```python
from build123d import *

# Parameters (mm, degrees)
SKETCH1_W            = 130
SKETCH1_H            = 156
SKETCH1_R            = 3
BOSS_EXTRUDE1_DEPTH  = 10
SKETCH2_R            = 2.5
CUT_EXTRUDE1_DEPTH   = 10
SKETCH3_W            = 130
SKETCH3_H            = 10
BOSS_EXTRUDE2_DEPTH  = 10
SKETCH4_W            = 130
SKETCH4_H            = 10
BOSS_EXTRUDE3_DEPTH  = 10
SKETCH5_W            = 130
SKETCH5_H            = 10
CUT_EXTRUDE2_DEPTH   = 12.25
SKETCH6_W            = 130
SKETCH6_H            = 12.25
CUT_EXTRUDE3_DEPTH   = 20
SKETCH7_W            = 130
SKETCH7_H            = 10
BOSS_EXTRUDE5_DEPTH  = 2.25
SKETCH8_W            = 130
SKETCH8_H            = 10
BOSS_EXTRUDE6_DEPTH  = 2.25
SKETCH10_W           = 130
SKETCH10_H           = 10
BOSS_EXTRUDE8_DEPTH  = 10
SKETCH11_W           = 130
SKETCH11_H           = 10
BOSS_EXTRUDE10_DEPTH = 7
SKETCH12_W           = 130
SKETCH12_H           = 10
CUT_EXTRUDE4_DEPTH   = 7
SKETCH14_W           = 130
SKETCH14_H           = 10
CUT_EXTRUDE5_DEPTH   = 10


with BuildPart() as part:
    # Sketch1 → Boss-Extrude1 (new body)
    with BuildSketch(Plane(origin=(0, 0, 0), x_dir=(1, 0, 0), z_dir=(0, 1, 0))):
        with Locations((65, -43.506875339)):
            Rectangle(SKETCH1_W, SKETCH1_H)
        with Locations(Location((5, 27.493124661, 0), (0, 0, 270))):
            Circle(SKETCH1_R, mode=Mode.SUBTRACT)
        with Locations(Location((45, 27.493124661, 0), (0, 0, 270))):
            Circle(SKETCH1_R, mode=Mode.SUBTRACT)
        with Locations(Location((45, -12.506875339, 0), (0, 0, 270))):
            Circle(SKETCH1_R, mode=Mode.SUBTRACT)
        with Locations(Location((5, -12.506875339, 0), (0, 0, 270))):
            Circle(SKETCH1_R, mode=Mode.SUBTRACT)
        with Locations(Location((85, 27.493124661, 0), (0, 0, 270))):
            Circle(SKETCH1_R, mode=Mode.SUBTRACT)
        with Locations(Location((125, 27.493124661, 0), (0, 0, 270))):
            Circle(SKETCH1_R, mode=Mode.SUBTRACT)
        with Locations(Location((85, -12.506875339, 0), (0, 0, 270))):
            Circle(SKETCH1_R, mode=Mode.SUBTRACT)
        with Locations(Location((125, -12.506875339, 0), (0, 0, 270))):
            Circle(SKETCH1_R, mode=Mode.SUBTRACT)
        with Locations(Location((85, -74.506875339, 0), (0, 0, 270))):
            Circle(SKETCH1_R, mode=Mode.SUBTRACT)
        with Locations(Location((125, -74.506875339, 0), (0, 0, 270))):
            Circle(SKETCH1_R, mode=Mode.SUBTRACT)
        with Locations(Location((125, -114.506875339, 0), (0, 0, 270))):
            Circle(SKETCH1_R, mode=Mode.SUBTRACT)
        with Locations(Location((85, -114.506875339, 0), (0, 0, 270))):
            Circle(SKETCH1_R, mode=Mode.SUBTRACT)
        with Locations(Location((5, -74.506875339, 0), (0, 0, 270))):
            Circle(SKETCH1_R, mode=Mode.SUBTRACT)
        with Locations(Location((45, -74.506875339, 0), (0, 0, 270))):
            Circle(SKETCH1_R, mode=Mode.SUBTRACT)
        with Locations(Location((5, -114.506875339, 0), (0, 0, 270))):
            Circle(SKETCH1_R, mode=Mode.SUBTRACT)
        with Locations(Location((45, -114.506875339, 0), (0, 0, 270))):
            Circle(SKETCH1_R, mode=Mode.SUBTRACT)
    extrude(amount=BOSS_EXTRUDE1_DEPTH)

    # Sketch2 → Cut-Extrude1 (cut)
    with BuildSketch(Plane(origin=(0, 10, 0), x_dir=(1, 0, 0), z_dir=(0, 1, 0))):
        with Locations(Location((98, -31.506875339, 0), (0, 0, 270))):
            Circle(SKETCH2_R)
        with Locations(Location((98, -55.506875339, 0), (0, 0, 270))):
            Circle(SKETCH2_R)
        with Locations(Location((122, -55.506875339, 0), (0, 0, 270))):
            Circle(SKETCH2_R)
        with Locations(Location((122, -31.506875339, 0), (0, 0, 270))):
            Circle(SKETCH2_R)
    extrude(amount=-CUT_EXTRUDE1_DEPTH, mode=Mode.SUBTRACT)

    # Sketch3 → Boss-Extrude2 (add)
    with BuildSketch(Plane(origin=(0, 0, -34.493124661), x_dir=(-1, 0, 0), z_dir=(0, 0, -1))):
        with Locations((-65, 5)):
            Rectangle(SKETCH3_W, SKETCH3_H)
    extrude(amount=BOSS_EXTRUDE2_DEPTH)

    # Sketch4 → Boss-Extrude3 (add)
    with BuildSketch(Plane.XY.offset(121.506875339)):
        with Locations((65, 5)):
            Rectangle(SKETCH4_W, SKETCH4_H)
    extrude(amount=BOSS_EXTRUDE3_DEPTH)

    # Sketch5 → Cut-Extrude2 (cut)
    with BuildSketch(Plane.XY.offset(131.506875339)):
        with Locations((65, 5)):
            Rectangle(SKETCH5_W, SKETCH5_H)
    extrude(amount=-CUT_EXTRUDE2_DEPTH, mode=Mode.SUBTRACT)

    # Sketch6 → Cut-Extrude3 (cut)
    with BuildSketch(Plane(origin=(0, 10, 0), x_dir=(1, 0, 0), z_dir=(0, 1, 0))):
        with Locations((65, 38.368124661)):
            Rectangle(SKETCH6_W, SKETCH6_H)
    extrude(amount=-CUT_EXTRUDE3_DEPTH, mode=Mode.SUBTRACT)

    # Sketch7 → Boss-Extrude5 (add)
    with BuildSketch(Plane(origin=(0, 0, -32.243124661), x_dir=(-1, 0, 0), z_dir=(0, 0, -1))):
        with Locations((-65, 5)):
            Rectangle(SKETCH7_W, SKETCH7_H)
    extrude(amount=BOSS_EXTRUDE5_DEPTH)

    # Sketch8 → Boss-Extrude6 (add)
    with BuildSketch(Plane.XY.offset(119.256875339)):
        with Locations((65, 5)):
            Rectangle(SKETCH8_W, SKETCH8_H)
    extrude(amount=BOSS_EXTRUDE6_DEPTH)

    # Sketch10 → Boss-Extrude8 (add)
    with BuildSketch(Plane.XY.offset(121.506875339)):
        with Locations((65, 5)):
            Rectangle(SKETCH10_W, SKETCH10_H)
    extrude(amount=BOSS_EXTRUDE8_DEPTH)

    # Sketch11 → Boss-Extrude10 (add)
    with BuildSketch(Plane(origin=(0, 0, -34.493124661), x_dir=(-1, 0, 0), z_dir=(0, 0, -1))):
        with Locations((-65, 5)):
            Rectangle(SKETCH11_W, SKETCH11_H)
    extrude(amount=BOSS_EXTRUDE10_DEPTH)

    # Sketch12 → Cut-Extrude4 (cut)
    with BuildSketch(Plane(origin=(0, 0, -41.493124661), x_dir=(-1, 0, 0), z_dir=(0, 0, -1))):
        with Locations((-65, 5)):
            Rectangle(SKETCH12_W, SKETCH12_H)
    extrude(amount=-CUT_EXTRUDE4_DEPTH, mode=Mode.SUBTRACT)

    # Sketch14 → Cut-Extrude5 (cut)
    with BuildSketch(Plane.XY.offset(131.506875339)):
        with Locations((65, 5)):
            Rectangle(SKETCH14_W, SKETCH14_H)
    extrude(amount=-CUT_EXTRUDE5_DEPTH, mode=Mode.SUBTRACT)


solid = part.part
```
Design review of the part built by this model. Coordinates are the model's own, in mm. Coordinates: 2 decimals unless noted, no trailing zeros. Write each loop counter-clockwise with the first axis right and the second up, starting at its lowest first coordinate (ties: lowest second). Pieces come first, ordered by that corner, then holes.
1) Mouldability with a two-part tool opening along X and no side actions: class faces 1 (the flat face through (130, 5, 45)), 2 (the flat face through (0, 5, 45)), 3 (the flat face through (66, 10, 45)), 4 (the cylindrical face through (127.974, 4.93, -27.884)) as +X half, -X half, draft (parallel to the pull), parting line (faces both ways), or undercut.
2) Add section C-C (x = 85). Write out the cut boundary in (y, z), plus the area to 3 significant figures.
3) Add section A-A (x = 98). Write out the cut boundary in (y, z).
4) Add section B-B (y = 2). State how many separate pieces and enclosed holes the cut face has, plus the area to 3 significant figures.
5) Insertion check: pin 1 (5.5 mm diameter, centred on x = 5, z = -27.49, fed in from +Y). The pin has a flat end and moves straight along its axis. Give the tip position at first contact, or say it passes through.
6) To check wall thickness, follow L1, parallel to X at y = 7.25, z = -27; L2, parallel to X at y = 7.75, z = 15; L3, parallel to X at y = 7.75, z = 54.5. State the ranges of each line that lie inside material, in increasing order.
Check result:
1. face 1: +X half
1. face 2: -X half
1. face 3: draft
1. face 4: undercut
2. outline: (0, -34.49) - (10, -34.49) - (10, -30.49) - (0, -30.49) - close; (0, -24.49) - (10, -24.49) - (10, 9.51) - (0, 9.51) - close; (0, 15.51) - (10, 15.51) - (10, 71.51) - (0, 71.51) - close; (0, 77.51) - (10, 77.51) - (10, 111.51) - (0, 111.51) - close; (0, 117.51) - (10, 117.51) - (10, 121.51) - (0, 121.51) - close
2. area: 1,320 mm2
3. outline: (0, -34.49) - (10, -34.49) - (10, 29.01) - (0, 29.01) - close; (0, 34.01) - (10, 34.01) - (10, 53.01) - (0, 53.01) - close; (0, 58.01) - (10, 58.01) - (10, 121.51) - (0, 121.51) - close
4. separate pieces: 1
4. enclosed holes: 20
4. area: 19,700 mm2
5. pin 1: passes through
6. L1: x = 0 to 2.04, 7.96 to 42.04, 47.96 to 82.04, 87.96 to 122.04, 127.96 to 130
6. L2: x = 0 to 3.33, 6.67 to 43.33, 46.67 to 83.33, 86.67 to 123.33, 126.67 to 130
6. L3: x = 0 to 95.71, 100.29 to 119.71, 124.29 to 130
